from build123d import *

# Parameters (mm, degrees)
BOSS_EXTRUDE1_DEPTH     = 31.75
SHELL1_T                = -6
FILLET1_R               = 5.334
CUT_EXTRUDE1_DEPTH      = 1.2954
FILLET2_R               = 0.254
FILLET3_R               = 0.127
BOSS_EXTRUDE2_DEPTH     = 12
SKETCH4_R               = 3.025
CUT_EXTRUDE2_DEPTH      = 9
MIRROR2_COPY_1_DEPTH    = 12
MIRROR2_COPY_2_SKETCH_R = 3.025
MIRROR2_COPY_2_DEPTH    = 9
CUT_EXTRUDE3_DEPTH      = 6
CUT_EXTRUDE4_START      = -3
SKETCH7_R               = 11.43
SKETCH7_R_2             = 6.35
CUT_EXTRUDE4_DEPTH      = 3


with BuildPart() as part:
    # Sketch1 → Boss-Extrude1 (new, symmetric)
    with BuildSketch(Plane.XY):
        Polygon((-34, -37), (-34, -16.68), (-34, 16.68), (-34, 37), (34, 37), (34, -37), align=None)
    extrude(amount=BOSS_EXTRUDE1_DEPTH, both=True)

    # Shell1
    shell1_openings = [part.faces().sort_by_distance(p)[0] for p in [
        (0, 0, 31.75),
    ]]
    offset(amount=SHELL1_T, openings=shell1_openings, kind=Kind.INTERSECTION)

    # Fillet1
    fillet1_edges = [part.edges().sort_by_distance(p)[0] for p in [
        (-34, -37, 0),
        (-34, 37, 0),
        (34, 37, 0),
        (34, -37, 0),
        (-28, -31, 3),
        (28, -31, 3),
        (28, 31, 3),
        (-28, 31, 3),
    ]]
    fillet(fillet1_edges, radius=FILLET1_R)

    # Sketch2 → Cut-Extrude1 (cut)
    with BuildSketch(Plane.XY.offset(31.75)):
        with BuildLine():
            Line((32.2827, -25.666), (32.2827, 25.666))
            ThreePointArc((32.2827, 25.666), (29.466033783, 32.466033783), (22.666, 35.2827))
            Line((22.666, 35.2827), (-22.666, 35.2827))
            ThreePointArc((-22.666, 35.2827), (-29.466033783, 32.466033783), (-32.2827, 25.666))
            Line((-32.2827, 25.666), (-32.2827, -25.666))
            ThreePointArc((-32.2827, -25.666), (-29.466033783, -32.466033783), (-22.666, -35.2827))
            Line((-22.666, -35.2827), (22.666, -35.2827))
            ThreePointArc((22.666, -35.2827), (29.466033783, -32.466033783), (32.2827, -25.666))
        make_face()
        with BuildLine():
            Line((-29.7173, 25.666), (-29.7173, -25.666))
            ThreePointArc((-29.7173, -25.666), (-27.652022046, -30.652022046), (-22.666, -32.7173))
            Line((-22.666, -32.7173), (22.666, -32.7173))
            ThreePointArc((22.666, -32.7173), (27.652022046, -30.652022046), (29.7173, -25.666))
            Line((29.7173, -25.666), (29.7173, 25.666))
            ThreePointArc((29.7173, 25.666), (27.652022046, 30.652022046), (22.666, 32.7173))
            Line((22.666, 32.7173), (-22.666, 32.7173))
            ThreePointArc((-22.666, 32.7173), (-27.652022046, 30.652022046), (-29.7173, 25.666))
        make_face(mode=Mode.SUBTRACT)
    extrude(amount=-CUT_EXTRUDE1_DEPTH, mode=Mode.SUBTRACT)

    # Fillet2
    fillet2_edges = [part.edges().sort_by_distance(p)[0] for p in [
        (29.466033783, -32.466033783, 30.4546),
        (0, -35.2827, 30.4546),
        (-29.466033783, -32.466033783, 30.4546),
        (-32.2827, 0, 30.4546),
        (-29.466033783, 32.466033783, 30.4546),
        (0, 35.2827, 30.4546),
        (29.466033783, 32.466033783, 30.4546),
        (32.2827, 0, 30.4546),
        (0, 32.7173, 30.4546),
        (-27.652022046, 30.652022046, 30.4546),
        (-29.7173, 0, 30.4546),
        (-27.652022046, -30.652022046, 30.4546),
        (0, -32.7173, 30.4546),
        (27.652022046, -30.652022046, 30.4546),
        (29.7173, 0, 30.4546),
        (27.652022046, 30.652022046, 30.4546),
    ]]
    fillet(fillet2_edges, radius=FILLET2_R)

    # Fillet3
    fillet3_edges = [part.edges().sort_by_distance(p)[0] for p in [
        (29.466033783, -32.466033783, 31.75),
        (32.2827, 0, 31.75),
        (29.466033783, 32.466033783, 31.75),
        (0, 35.2827, 31.75),
        (-29.466033783, 32.466033783, 31.75),
        (-32.2827, 0, 31.75),
        (-29.466033783, -32.466033783, 31.75),
        (0, -35.2827, 31.75),
        (-27.652022046, 30.652022046, 31.75),
        (0, 32.7173, 31.75),
        (27.652022046, 30.652022046, 31.75),
        (29.7173, 0, 31.75),
        (27.652022046, -30.652022046, 31.75),
        (0, -32.7173, 31.75),
        (-27.652022046, -30.652022046, 31.75),
        (-29.7173, 0, 31.75),
    ]]
    fillet(fillet3_edges, radius=FILLET3_R)

    # Sketch3 → Boss-Extrude2 (add)
    with BuildSketch(Plane.XY.offset(31.75)):
        with BuildLine():
            Line((34, -29.221825407), (34, -31.666))
            ThreePointArc((34, -31.666), (32.437707571, -35.437707571), (28.666, -37))
            Line((28.666, -37), (26.221825407, -37))
            Line((26.221825407, -37), (29.202282953, -39.980457546))
            ThreePointArc((29.202282953, -39.980457546), (36.980457546, -39.980457546), (36.980457546, -32.202282953))
            Line((36.980457546, -32.202282953), (34, -29.221825407))
        make_face()
    boss_extrude2 = extrude(amount=-BOSS_EXTRUDE2_DEPTH)

    # Sketch4 → Cut-Extrude2 (cut)
    with BuildSketch(Plane.XY.offset(31.75)):
        with Locations((33.09137025, -36.09137025)):
            Circle(SKETCH4_R)
    cut_extrude2 = extrude(amount=-CUT_EXTRUDE2_DEPTH, mode=Mode.SUBTRACT)

    # Mirror1: Boss-Extrude2, Cut-Extrude2 across plane
    add(boss_extrude2.mirror(Plane.ZX))
    add(cut_extrude2.mirror(Plane.ZX), mode=Mode.SUBTRACT)

    # Mirror2: Boss-Extrude2, Cut-Extrude2 across plane
    add(boss_extrude2.mirror(Plane(origin=(0, 0, 0), x_dir=(0, 0, 1), z_dir=(1, 0, 0))))
    add(cut_extrude2.mirror(Plane(origin=(0, 0, 0), x_dir=(0, 0, 1), z_dir=(1, 0, 0))), mode=Mode.SUBTRACT)

    # Mirror2 copy 1 sketch → Mirror2 copy 1 (add)
    with BuildSketch(Plane(origin=(0, 0, 31.75), x_dir=(-1, 0, 0), z_dir=(0, 0, 1))):
        with BuildLine():
            Line((34, -29.221825407), (34, -31.666))
            ThreePointArc((34, -31.666), (32.437707571, -35.437707571), (28.666, -37))
            Line((28.666, -37), (26.221825407, -37))
            Line((26.221825407, -37), (29.202282953, -39.980457546))
            ThreePointArc((29.202282953, -39.980457546), (36.980457546, -39.980457546), (36.980457546, -32.202282953))
            Line((36.980457546, -32.202282953), (34, -29.221825407))
        make_face()
    extrude(amount=-MIRROR2_COPY_1_DEPTH)

    # Mirror2 copy 2 sketch → Mirror2 copy 2 (cut)
    with BuildSketch(Plane(origin=(0, 0, 31.75), x_dir=(-1, 0, 0), z_dir=(0, 0, 1))):
        with Locations((33.09137025, -36.09137025)):
            Circle(MIRROR2_COPY_2_SKETCH_R)
    extrude(amount=-MIRROR2_COPY_2_DEPTH, mode=Mode.SUBTRACT)

    # Sketch6 → Cut-Extrude3 (cut)
    with BuildSketch(Plane(origin=(0, 37, 0), x_dir=(1, 0, 0), z_dir=(0, 1, 0))):
        with BuildLine():
            ThreePointArc((0, 6.35), (-6.35, 0), (0, -6.35))
            Line((0, -6.35), (0, 6.35))
        make_face()
        with BuildLine():
            Line((0, 6.35), (0, -6.35))
            ThreePointArc((0, -6.35), (4.490128061, -4.490128061), (6.35, 0))
            ThreePointArc((6.35, 0), (4.490128061, 4.490128061), (0, 6.35))
        make_face()
    extrude(amount=-CUT_EXTRUDE3_DEPTH, mode=Mode.SUBTRACT)

    # Sketch7 → Cut-Extrude4 (cut)
    with BuildSketch(Plane.XZ.offset(-31).offset(CUT_EXTRUDE4_START)):
        Circle(SKETCH7_R)
        with Locations(Location((0, 0, 0), (0, 0, 180))):
            Circle(SKETCH7_R_2, mode=Mode.SUBTRACT)
    extrude(amount=CUT_EXTRUDE4_DEPTH, mode=Mode.SUBTRACT)


solid = part.part
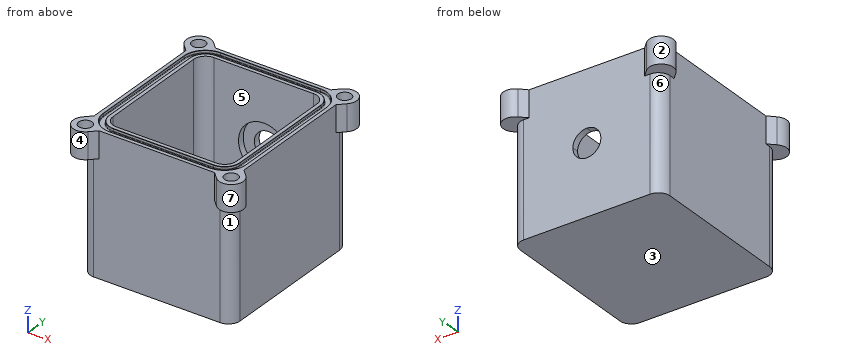
Can you work these out from the model? Positions are in its coordinate system, mm. Face numbers are marked on the shaded views. A direction names the side the tool comes from. Coordinates: 2 decimals unless noted, no trailing zeros. Write each loop counter-clockwise with the first axis right and the second up, starting at its lowest first coordinate (ties: lowest second). Pieces come first, ordered by that corner, then holes. Notation, with made-up numbers: (67, 47.5) - (98, 47.5) arc R4 cw to (98, 53.5) - close; hole circle Ø1 at (44.25, 83.25). An arc over 180 degrees is marked (long way). Return JSON: item names as keys, results as strings. Group by question number.
Item 1: Please list where these lines run through material, in increasing order: probe 1 along X at (y, z) = (2.5, 14.5); probe 2 along Y at (x, z) = (-5.5, -12); probe 3 along Z at (x, y) = (-21, -5.5).
Item 2: We'd pull the mould along Y, two halves only. Please class the marked faces 1, 2, 3 and 4: pulls with the +Y half, pulls with the -Y half, needs draft (parallel to the pull), parting line crosses it, or undercut.
Item 3: I'm going to push flat-ended pins straight in: pin 1 Ø13.5 at (x, y) = (32, -38) entering from -Z; pin 2 Ø5.5 at (x, y) = (-33.09, 36.09) entering from +Z; pin 3 Ø22.5 at (x, z) = (-4.5, 6) entering from +Y; pin 4 Ø12 at (y, z) = (2.5, 7.5) entering from +X. Where does each tip first touch, or does it pass through?
Item 4: If we section it at A-A (z = 12.5): Write out the boundary of the cut face in (x, y), then the cut area to 3 significant figures.
Item 5: Which directions (+Z, -Z, +X, -X, +Y, -Y) give clear straight access to the entire face, cutting with the end or side of a thin tool? Please do the marked faces 5, 6 and 7.
Item 6: If we section it at B-B (z = -27.5): Write out the boundary of the cut face in (x, y), then the cut area to 3 significant figures.
Item 7: If we section it at D-D (y = 8): Write out the boundary of the cut face in (x, z).
Item 8: If we section it at C-C (x = -20): Write out the boundary of the cut face in (y, z).
Return value:
{
 "1": {"probe 1": "x = -34 to -28, 28 to 34", "probe 2": "y = -37 to -31, 31 to 37", "probe 3": "z = -31.75 to -25.75"},
 "2": {"face 1": "pulls with the -Y half", "face 2": "undercut", "face 3": "needs draft", "face 4": "undercut"},
 "3": {"pin 1": "stops at z = -31.75", "pin 2": "stops at z = 22.75", "pin 3": "stops at y = 37", "pin 4": "stops at x = 34"},
 "4": {"outline": "(-34, -31.67) arc R5.33 ccw to (-28.67, -37) - (28.67, -37) arc R5.33 ccw to (34, -31.67) - (34, 31.67) arc R5.33 ccw to (28.67, 37) - (-28.67, 37) arc R5.33 ccw to (-34, 31.67) - close; hole (-28, -25.67) arc R5.33 ccw to (-22.67, -31) - (22.67, -31) arc R5.33 ccw to (28, -25.67) - (28, 25.67) arc R5.33 ccw to (22.67, 31) - (-22.67, 31) arc R5.33 ccw to (-28, 25.67) - close", "area": "1,560 mm^2"},
 "5": {"face 5": "+Z", "face 6": "-Z, -X, +Y", "face 7": "+Z, -Z"},
 "6": {"outline": "(-34, -31.67) arc R5.33 ccw to (-28.67, -37) - (28.67, -37) arc R5.33 ccw to (34, -31.67) - (34, 31.67) arc R5.33 ccw to (28.67, 37) - (-28.67, 37) arc R5.33 ccw to (-34, 31.67) - close", "area": "5,010 mm^2"},
 "7": {"outline": "(-34, -31.75) - (34, -31.75) - (34, 31.75) - (32.41, 31.75) arc R0.13 ccw to (32.28, 31.62) - (32.28, 30.71) arc R0.25 cw to (32.03, 30.45) - (29.97, 30.45) arc R0.25 cw to (29.72, 30.71) - (29.72, 31.62) arc R0.13 ccw to (29.59, 31.75) - (28, 31.75) - (28, -25.75) - (-28, -25.75) - (-28, 31.75) - (-29.59, 31.75) arc R0.13 ccw to (-29.72, 31.62) - (-29.72, 30.71) arc R0.25 cw to (-29.97, 30.45) - (-32.03, 30.45) arc R0.25 cw to (-32.28, 30.71) - (-32.28, 31.62) arc R0.13 ccw to (-32.41, 31.75) - (-34, 31.75) - close"},
 "8": {"outline": "(-37, -31.75) - (37, -31.75) - (37, 31.75) - (35.41, 31.75) arc R0.13 ccw to (35.28, 31.62) - (35.28, 30.71) arc R0.25 cw to (35.03, 30.45) - (32.97, 30.45) arc R0.25 cw to (32.72, 30.71) - (32.72, 31.62) arc R0.13 ccw to (32.59, 31.75) - (31, 31.75) - (31, -25.75) - (-31, -25.75) - (-31, 31.75) - (-32.59, 31.75) arc R0.13 ccw to (-32.72, 31.62) - (-32.72, 30.71) arc R0.25 cw to (-32.97, 30.45) - (-35.03, 30.45) arc R0.25 cw to (-35.28, 30.71) - (-35.28, 31.62) arc R0.13 ccw to (-35.41, 31.75) - (-37, 31.75) - close"}
}
